from build123d import *

# Parameters (mm, degrees)
F0_W     = 31.75
F0_H     = 63.4180661291
F1_DEPTH = 12.7
F2_R     = 5.5188922036
F3_T     = -1.27
F4_R     = 8.1477804886
F5_DEPTH = 2.4384


with BuildPart() as f1:
    # F0 (on Top) → F1 (new body)
    with BuildSketch(Plane.XY):
        with Locations((-0.6452417001, -7.6507264748)):
            Rectangle(F0_W, F0_H)
    extrude(amount=F1_DEPTH)

    # F2
    f2_edges = [f1.edges().sort_by_distance(p)[0] for p in [
        (-16.520242, -7.650726, 12.7),
        (-0.645242, -39.35976, 12.7),
        (15.229758, -7.650726, 12.7),
        (-0.645242, 24.058307, 12.7),
    ]]
    fillet(f2_edges, radius=F2_R)

    # F3
    f3_openings = [f1.faces().sort_by_distance(p)[0] for p in [
        (-0.645242, -7.650726, 0),
    ]]
    offset(amount=F3_T, openings=f3_openings)

    # F4 (on face) → F5 (join)
    with BuildSketch(Plane.XY.offset(12.7)):
        Circle(F4_R)
        with BuildLine():
            ThreePointArc((-0.7278024156, -7.0990652471), (-7.1362752006, 0), (-0.7278024156, 7.0990652471))
            Line((-0.7278024156, 7.0990652471), (-0.7278024156, -7.0990652471))
        make_face(mode=Mode.SUBTRACT)
        with BuildLine():
            Line((0.7278024156, -7.0990652471), (0.7113547333, 7.1007322285))
            ThreePointArc((0.7113547333, 7.1007322285), (7.1362704133, 0.0082659706), (0.7278024156, -7.0990652471))
        make_face(mode=Mode.SUBTRACT)
        with BuildLine():
            add(Edge.make_bspline(
                [(-4.9823397783, -1.5874156443), (-4.6270242199, -1.7415742797), (-3.9270228794, -2.0452796731), (-2.765918201, -2.34592671), (-2.2627830963, -1.941959242), (-2.0254463889, -1.7514014617)],
                knots=[0, 0, 0, 0, 0.3525731836, 0.6945986327, 1, 1, 1, 1], degree=3))
            Line((-2.0254463889, -1.7514014617), (-4.9851336516, 0.8246224024))
            Line((-4.9851336516, 0.8246224024), (-4.9823397783, -1.5874156443))
        make_face()
        with BuildLine():
            Line((4.9851336516, 0.8246224024), (2.0254463889, -1.7514014617))
            add(Edge.make_bspline(
                [(4.9823397783, -1.5874156443), (4.6270242199, -1.7415742797), (3.9270228794, -2.0452796731), (2.765918201, -2.34592671), (2.2627830963, -1.941959242), (2.0254463889, -1.7514014617)],
                knots=[0, 0, 0, 0, 0.3525731836, 0.6945986327, 1, 1, 1, 1], degree=3))
            Line((4.9823397783, -1.5874156443), (4.9851336516, 0.8246224024))
        make_face()
    extrude(amount=F5_DEPTH)


solid = f1.part
Source: CAD feature listing. Evaluate the final solid. Frame: model axes, mm. A direction names the side the tool comes from. Give positions to 0.01 mm unless a question says otherwise; leave off trailing zeros. Write each loop counter-clockwise with the first axis right and the second up, starting at its lowest first coordinate (ties: lowest second). Pieces come first, ordered by that corner, then holes. Notation, with made-up numbers: M 14,4.5 L 54,4.5 A33 ccw 54,37.5 Z; hole C 37,11 d7. An arc over 180 degrees is marked long. Return JSON: item names as keys, results as strings. Group by question number.
1) Cut plane C-C, the plane x = 9. Output: boundary loops of the cut face in (y, z).
2) Cut plane A-A, the plane z = 6. Output: boundary loops of the cut face in (x, y), then the cut area to 3 significant figures.
3) Ray query, L1, parallel to Y at x = -13, z = 7; L2, parallel to X at y = -6, z = 6.25; L3, parallel to Y at x = -7.5, z = 7.5. Return the intervals inside material, ascending.
4) Set-up query: faces 1 (the face through (-14.946, -7.207, 11.04)), 2 (the face through (-0.44, 21.58, 10.15)), 3 (the face through (3.526, -0.445, 13.902)). Return all of +Z, -Z, +X, -X, +Y, -Y with unobstructed straight access to the full face (end or side cutting, diameter ignored); none if empty.
5) First-contact query: pin 1 Ø3 at (y, z) = (-3, 8) entering from -X; pin 2 Ø2 at (x, z) = (-11.5, 10.5) entering from +Y; pin 3 Ø6 at (x, y) = (2, -8.5) entering from -Z; pin 4 Ø6 at (x, y) = (-0.5, -19.5) entering from +Z. Flat tips, straight axial feed; report the tip coordinate or a pass-through.
6) Draft query along Y for faces 4 (the face through (-0.423, -37.786, 11.04)), 5 (the face through (13.96, -8, 4)), 6 (the face through (-16.52, -8, 4)). Return one class per face: released by +Y, released by -Y, zero draft, split by the parting line, or undercut.
7) Cut plane B-B, the plane y = -13. Output: boundary loops of the cut face in (x, z).
8) Cut plane D-D, the plane x = 0. Output: boundary loops of the cut face in (y, z).
Data:
{
 "1": {"outline": "M -39.36,0 L -38.09,0 L -38.09,7.18 A4.25 cw -33.84,11.43 L 18.54,11.43 A4.25 cw 22.79,7.18 L 22.79,0 L 24.06,0 L 24.06,7.18 A5.52 ccw 18.54,12.7 L -33.84,12.7 A5.52 ccw -39.36,7.18 Z"},
 "2": {"outline": "M -16.52,-39.36 L 15.23,-39.36 L 15.23,24.06 L -16.52,24.06 Z; hole M -15.25,-38.09 L 13.96,-38.09 L 13.96,22.79 L -15.25,22.79 Z", "area": "235 mm²"},
 "3": {"L1": "y = -39.36 to -38.09, 22.79 to 24.06", "L2": "x = -16.52 to -15.25, 13.96 to 15.23", "L3": "y = -39.35 to -38.08, 22.78 to 24.05"},
 "4": {"face 1": "+Z, -X, +Y, -Y", "face 2": "-Z", "face 3": "+Z"},
 "5": {"pin 1": "stops at x = -16.52", "pin 2": "stops at y = 23.55", "pin 3": "stops at z = 11.43", "pin 4": "stops at z = 12.7"},
 "6": {"face 4": "released by -Y", "face 5": "undercut", "face 6": "zero draft"},
 "7": {"outline": "M -16.52,0 L -15.25,0 L -15.25,7.18 A4.25 cw -11,11.43 L 9.71,11.43 A4.25 cw 13.96,7.18 L 13.96,0 L 15.23,0 L 15.23,7.18 A5.52 ccw 9.71,12.7 L -11,12.7 A5.52 ccw -16.52,7.18 Z"},
 "8": {"outline": "M -39.36,0 L -38.09,0 L -38.09,7.18 A4.25 cw -33.84,11.43 L 18.54,11.43 A4.25 cw 22.79,7.18 L 22.79,0 L 24.06,0 L 24.06,7.18 A5.52 ccw 18.54,12.7 L 8.15,12.7 L 8.15,15.14 L -8.15,15.14 L -8.15,12.7 L -33.84,12.7 A5.52 ccw -39.36,7.18 Z"}
}
